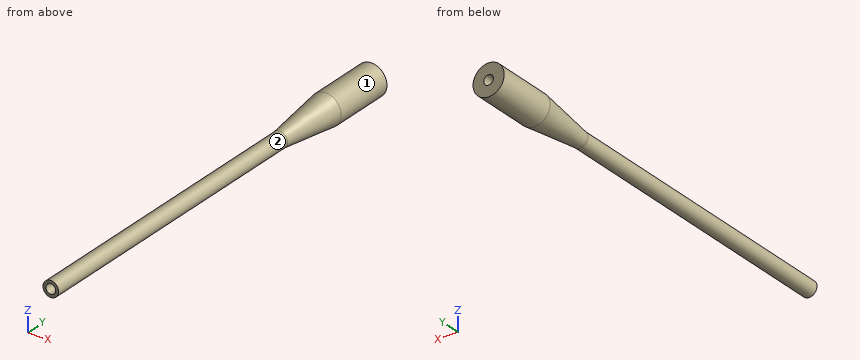
```python
from build123d import *

# Parameters (mm, degrees)
F0_R     = 6.35
F1_DEPTH = 254
F5_R     = 12.7
F6_DEPTH = 50.8
F4_R     = 12.7
F8_R     = 3.9116
F9_DEPTH = 406.4


with BuildPart() as f1:
    # F0 (on Front) → F1 (new body)
    with BuildSketch(Plane.XZ):
        Circle(F0_R)
    extrude(amount=F1_DEPTH)



with BuildPart() as f6:
    # F5 (on offset) → F6 (new body)
    with BuildSketch(Plane.XZ.offset(-101.6)):
        Circle(F5_R)
    extrude(amount=F6_DEPTH)


with BuildPart() as f1_1:
    add(f1.part)

    add(f6.part)  # F7 merges F6
    # F4 (on offset) → F7 section 0
    with BuildSketch(Plane.XZ.offset(-50.8)):
        Circle(F4_R)
    # F0 (on Front) → F7 section 1
    with BuildSketch(Plane.XZ):
        Circle(F0_R)
    loft()

    # F8 (on face) → F9 (cut)
    with BuildSketch(Plane.XZ.offset(-101.6)):
        Circle(F8_R)
    extrude(amount=F9_DEPTH, mode=Mode.SUBTRACT)


solid = f1_1.part
```
Work out the finished part from the listing and answer in its coordinate system (mm). Face numbers are marked on the shaded views. A direction names the side the tool comes from. Coordinates: 2 decimals unless noted, no trailing zeros. Write each loop counter-clockwise with the first axis right and the second up, starting at its lowest first coordinate (ties: lowest second). Pieces come first, ordered by that corner, then holes.
Q1. Which of the six approach directions +Z, -Z, +X, -X, +Y, -Y give full straight-line access (tool end or side, diameter ignored) to the marked faces 1 and 2?
Q2. Find the intervals of material crossed by line 1 (Z direction, x = 0, y = -116); line 2 (X direction, y = -11, z = -5); line 3 (X direction, y = 22.5, z = 0), in increasing order.
Q3. A cutting plane is placed at B-B, the plane y = -208. Give the vertices of the cut face in (x, z).
Q4. Each of these flat-tipped pins is pushed along its axis until it touches: pin 1 Ø5 at (y, z) = (-32.5, -7) entering from -X; pin 2 Ø4 at (x, y) = (7, -98.5) entering from +Z; pin 3 Ø1 at (x, y) = (-1, 14) entering from +Z; pin 4 Ø5 at (y, z) = (-27.5, -10) entering from -X. Where does it stop, or does it pass through?
Q5. A cutting plane is placed at A-A, the plane x = 0. Give the vertices of the cut face in (y, z), then the cut area to 3 significant figures.
Findings below:
1. face 1: +Y, -Y
1. face 2: -Y
2. line 1: z = -6.35 to -3.91, 3.91 to 6.35
2. line 2: x = -3.91 to 3.91
2. line 3: x = -9.16 to -3.91, 3.91 to 9.16
3. outline: circle Ø12.7 at (0, 0); hole circle Ø7.82 at (0, 0)
4. pin 1: stops at x = -4.48
4. pin 2: stops at z = 3.91
4. pin 3: stops at z = 8.12
4. pin 4: passes through
5. outline: (-254, -6.35) - (0, -6.35) - (50.8, -12.7) - (101.6, -12.7) - (101.6, -3.91) - (-254, -3.91) - close; (-254, 3.91) - (101.6, 3.91) - (101.6, 12.7) - (50.8, 12.7) - (0, 6.35) - (-254, 6.35) - close
5. area: 2,700 mm2
